Autodesk Inventor part; units mm, degrees
ref_plane "YZ Plane" through (0, 0, 0) normal (1, 0, 0) x (0, 1, 0)
ref_plane "XZ Plane" through (0, 0, 0) normal (0, 1, 0) x (-1, 0, 0)
ref_plane "XY Plane" through (0, 0, 0) normal (0, 0, 1) x (1, 0, 0)
sketch "Sketch1" plane through (0, 0, 0) normal (0, 0, 1) x (1, 0, 0)
  arc A0 (270.3829, -151.3678) -> (288.8718, 134.8752) centre (135.9788, 1.0322) ccw
  line L0 (358.2288, 204.2322) -> (358.2288, -202.1678)
  line L1 (358.2288, -202.1678) -> (147.3998, -202.1678)
  line L2 (147.3998, 204.2322) -> (553.7998, 204.2322) construction
  arc A1 (147.3998, -201.8466) -> (288.8718, 134.8752) centre (135.9788, 1.0322) ccw
  line L3 (147.3998, -201.8466) -> (147.3998, -202.1678)
  line L4 (358.2288, 204.2322) -> (288.8718, 134.8752)
  line L5 (358.2288, 204.2322) -> (456.3143, 204.2322) construction
  point P0 (270.3829, 153.4322)
  dimension "d5" = 203.2
  dimension "d9" = 135
extrude "Extrusion1" add sketch "Sketch1" along normal blind 12.7
sketch "Sketch2" plane through (0, 0, 0) normal (0, 0, -1) x (-1, 0, 0)
  line L0 (-358.2288, -202.1678) -> (-358.2288, 204.2322)
  line L1 (-147.3998, -202.1678) -> (-358.2288, -202.1678)
  point P0 (0, 0)
  point P1 (-288.3788, -161.5278)
  point P2 (-341.7188, -68.8178)
  point P3 (-331.5588, 122.9522)
  dimension "d10" = 69.85
  dimension "d11" = 40.64
  dimension "d12" = 16.51
  dimension "d13" = 133.35
  dimension "d14" = 325.12
  dimension "d15" = 26.67
hole "Hole1" at (288.3788, -161.5278, 0) at (341.7188, -68.8178, 0) at (331.5588, 122.9522, 0) direction (0, 0, 1) diameter 6.7564 end through all
properties part number "Hood (inside)" material "Wood (Oak)"
Geometry: final body of the model. Coordinates: model frame, mm. Give positions to 0.01 mm unless a question says otherwise; leave off trailing zeros. Order: outer loops, then holes, each group sorted by start corner. A loop starts at its lowest first (then second) coordinate and runs counter-clockwise, first axis right, second up. Notation, with made-up numbers: (50.25, 78) - (88.25, 78) arc R19 cw to (88.25, 89) - close; hole circle Ø7 at (-18.5, 9.25). An arc over 180 degrees is marked (long way). Use CSV: the item, a comma, the result in double quotes.
1. Section query A-A (x = 304.5). Output: boundary loops of the cut face in (y, z), plus the area to 3 significant figures.
Answers below:
outline,"(-202.17, 0) - (-112.51, 0) - (-112.51, 12.7) - (-202.17, 12.7) - close; (114.57, 0) - (150.5, 0) - (150.5, 12.7) - (114.57, 12.7) - close"
area,"1,600 mm2"
2. Mould query, pull axis Y, two halves, no side actions, for faces 1 (the face through (254, -202.168, 6)), 2 (the face through (338.888, -9.84, 6.261)), 3 (the face through (324.036, 170.039, 6.261)). Classes: +Y half, -Y half, draft (parallel to the pull), parting line (faces both ways), or undercut.
Answers below:
face 1,"-Y half"
face 2,"undercut"
face 3,"+Y half"
3. Section query D-D (x = 219). Output: boundary loops of the cut face in (y, z).
Answers below:
outline,"(-202.17, 0) - (-184.43, 0) - (-184.43, 12.7) - (-202.17, 12.7) - close"
4. Section query B-B (z = 4). Output: boundary loops of the cut face in (x, y).
Answers below:
outline,"(147.4, -202.17) - (358.23, -202.17) - (358.23, 204.23) - (288.87, 134.88) arc R203.2 cw to (270.38, -151.37) arc R203.2 cw to (147.4, -201.85) - close; hole circle Ø6.76 at (288.38, -161.53); hole circle Ø6.76 at (331.56, 122.95); hole circle Ø6.76 at (341.72, -68.82)"
5. Section query C-C (y = -22). Output: boundary loops of the cut face in (x, z).
Answers below:
outline,"(337.87, 0) - (358.23, 0) - (358.23, 12.7) - (337.87, 12.7) - close"
6. Material intervals for line 1 along X through (y, z) = (-1.5, 4.75); line 2 along Y through (x, z) = (291, 11.5); line 3 along Y through (x, z) = (313, 4.25), sorted ascending. Write a range as from..to.
Answers below:
line 1,"339.16..358.23"
line 2,"-202.17..-163.66, -159.4..-130.34, 132.4..137"
line 3,"-202.17..-98.74, 100.8..159"
7. Contact query for flat-ended pins moving along their axis: pin 1 (8 mm diameter, centred on x = 331.56, y = 122.95, fed in from +Z); pin 2 (6 mm diameter, centred on y = 132, z = 5.5, fed in from -X). Output: stop coordinate, or through.
Answers below:
pin 1,"z = 12.7"
pin 2,"x = 288.87"
